from build123d import *

# Parameters (mm, degrees)
SKETCH3_R           = 73.025
BOSS_EXTRUDE2_DEPTH = 3.175
SKETCH5_R           = 31.75
CUT_EXTRUDE3_DEPTH  = 7.35
CUT_EXTRUDE4_DEPTH  = 7.35
SKETCH7_3_R         = 12.7
BOSS_EXTRUDE4_DEPTH = 3.175


with BuildPart() as part:
    # Sketch3 → Boss-Extrude2 (new body, symmetric)
    with BuildSketch(Plane.XY):
        Circle(SKETCH3_R)
    extrude(amount=BOSS_EXTRUDE2_DEPTH, both=True)

    # Sketch5 → Cut-Extrude3 (cut, through all)
    with BuildSketch(Plane.XY.offset(3.175)):
        with Locations((92.075, 0)):
            Circle(SKETCH5_R)
        with Locations((46.0375, -79.739289053)):
            Circle(SKETCH5_R)
        with Locations((-46.0375, -79.739289053)):
            Circle(SKETCH5_R)
        with Locations((-92.075, 0)):
            Circle(SKETCH5_R)
        with Locations((-46.0375, 79.739289053)):
            Circle(SKETCH5_R)
        with Locations((46.0375, 79.739289053)):
            Circle(SKETCH5_R)
        with BuildLine():
            Line((66.176953095, 30.874933265), (36.170567884, 13.550738686))
            ThreePointArc((36.170567884, 13.550738686), (27.49630657, 15.875), (29.820567884, 24.549261314))
            Line((29.820567884, 24.549261314), (59.826953095, 41.873455893))
            ThreePointArc((59.826953095, 41.873455893), (68.501214409, 39.549194579), (66.176953095, 30.874933265))
        make_face()
        with BuildLine():
            Line((59.826953095, -41.873455893), (29.820567884, -24.549261314))
            ThreePointArc((29.820567884, -24.549261314), (27.49630657, -15.875), (36.170567884, -13.550738686))
            Line((36.170567884, -13.550738686), (66.176953095, -30.874933265))
            ThreePointArc((66.176953095, -30.874933265), (68.501214409, -39.549194579), (59.826953095, -41.873455893))
        make_face()
        with BuildLine():
            Line((-6.35, -72.748389157), (-6.35, -38.1))
            ThreePointArc((-6.35, -38.1), (0, -31.75), (6.35, -38.1))
            Line((6.35, -38.1), (6.35, -72.748389157))
            ThreePointArc((6.35, -72.748389157), (0, -79.098389157), (-6.35, -72.748389157))
        make_face()
        with BuildLine():
            Line((-66.176953095, -30.874933265), (-36.170567884, -13.550738686))
            ThreePointArc((-36.170567884, -13.550738686), (-27.49630657, -15.875), (-29.820567884, -24.549261314))
            Line((-29.820567884, -24.549261314), (-59.826953095, -41.873455893))
            ThreePointArc((-59.826953095, -41.873455893), (-68.501214409, -39.549194579), (-66.176953095, -30.874933265))
        make_face()
        with BuildLine():
            Line((-59.826953095, 41.873455893), (-29.820567884, 24.549261314))
            ThreePointArc((-29.820567884, 24.549261314), (-27.49630657, 15.875), (-36.170567884, 13.550738686))
            Line((-36.170567884, 13.550738686), (-66.176953095, 30.874933265))
            ThreePointArc((-66.176953095, 30.874933265), (-68.501214409, 39.549194579), (-59.826953095, 41.873455893))
        make_face()
        with BuildLine():
            Line((6.35, 72.748389157), (6.35, 38.1))
            ThreePointArc((6.35, 38.1), (0, 31.75), (-6.35, 38.1))
            Line((-6.35, 38.1), (-6.35, 72.748389157))
            ThreePointArc((-6.35, 72.748389157), (0, 79.098389157), (6.35, 72.748389157))
        make_face()
    extrude(amount=-CUT_EXTRUDE3_DEPTH, mode=Mode.SUBTRACT)

    # Sketch7 → Cut-Extrude4 (cut, through all)
    with BuildSketch(Plane.XY.offset(3.175)):
        with BuildLine():
            Line((6.148361062, 1.5875), (7.735861062, 1.5875))
            Line((7.735861062, 1.5875), (7.735861062, -1.5875))
            Line((7.735861062, -1.5875), (6.148361062, -1.5875))
            ThreePointArc((6.148361062, -1.5875), (-6.35, 0), (6.148361062, 1.5875))
        make_face()
    extrude(amount=-CUT_EXTRUDE4_DEPTH, mode=Mode.SUBTRACT)

    # Sketch7_3 → Boss-Extrude4 (add)
    with BuildSketch(Plane.XY.offset(3.175)):
        Circle(SKETCH7_3_R)
        with BuildLine():
            Line((6.148361062, 1.5875), (7.735861062, 1.5875))
            Line((7.735861062, 1.5875), (7.735861062, -1.5875))
            Line((7.735861062, -1.5875), (6.148361062, -1.5875))
            ThreePointArc((6.148361062, -1.5875), (-6.35, 0), (6.148361062, 1.5875))
        make_face(mode=Mode.SUBTRACT)
    extrude(amount=BOSS_EXTRUDE4_DEPTH)


solid = part.part
Geometry check sheet. Reference: the model listing, model coordinates, mm. A direction names the side the tool comes from. Round coordinates to 2 decimals unless told otherwise and drop trailing zeros. Loops run counter-clockwise (first coordinate to the right, second up) from the corner with the lowest first, then second, coordinate; pieces in that order, holes last. Notation, with made-up numbers: (2.5, -19) -> (9.5, -19) arc R33 ccw to (9.5, 15) -> close; hole circle Ø7 at (19, -22). An arc over 180 degrees is marked (long way). Answer as a JSON object with one key per item and string values. Group by question number.
Item 1: Cross-section at D-D, the plane y = -54. Record the cut outline in (x, z) (3 decimals), plus the area to 3 significant figures.
Item 2: Release check for a two-part mould opening along X. For faces 4 (the face through (6.35, 56, 0)), 5 (the face through (10.964, 72.197, 0.044)), 6 (the face through (-57.043, 45.593, 0.044)) record: pulls with the +X half, pulls with the -X half, needs draft (parallel to the pull), parting line crosses it, or undercut.
Item 3: Thickness scan on line 1 along X through (y, z) = (0, 3) (3 decimals); line 2 along Y through (x, z) = (-51, 0); line 3 along Y through (x, z) = (-47, 1.75). Record the ranges inside material, lowest first.
Item 4: Set-up check for faces 1 (the face through (6.35, -55, 0)), 2 (the face through (-6.35, 55, 0)), 3 (the face through (45.03, -33.33, 0.04)): record each of +Z, -Z, +X, -X, +Y, -Y from which the full face is reachable in a straight line by a thin tool's end or side.
Item 5: Cross-section at C-C, the plane x = -38.5. Record the cut outline in (y, z) (3 decimals), plus the area to 3 significant figures.
Item 6: Depth check by flat-ended pin: pin 1 Ø4 at (y, z) = (14.5, 4.5) entering from -X; pin 2 Ø3 at (y, z) = (53, -1) entering from -X; pin 3 Ø4 at (x, z) = (40, 4.5) entering from +Y; pin 4 Ø11.5 at (x, y) = (0, 0) entering from +Z. Enter the tip coordinate at first touch or a pass-through.
Item 7: Cross-section at B-B, the plane y = -19.05. Record the cut outline in (x, z) (3 decimals), plus the area to 3 significant figures.
Item 8: Cross-section at A-A, the plane x = 0. Record the cut outline in (y, z) (3 decimals).
Determined:
{
 "1": {"outline": "(-27.448, -3.175) -> (-6.35, -3.175) -> (-6.35, 3.175) -> (-27.448, 3.175) -> close; (6.35, -3.175) -> (27.448, -3.175) -> (27.448, 3.175) -> (6.35, 3.175) -> close", "area": "268 mm²"},
 "2": {"face 4": "undercut", "face 5": "pulls with the +X half", "face 6": "pulls with the -X half"},
 "3": {"line 1": "x = -60.325 to -6.35, 7.736 to 60.325", "line 2": "y = -48.38 to -36.78, -22.11 to 22.11, 36.78 to 48.38", "line 3": "y = -48 to -34.47, -19.8 to 19.8, 34.47 to 48"},
 "4": {"face 1": "+Z, -Z, -Y", "face 2": "+Z, -Z, +Y", "face 3": "+Z, -Z"},
 "5": {"outline": "(-48.897, -3.175) -> (-29.56, -3.175) -> (-29.56, 3.175) -> (-48.897, 3.175) -> close; (-14.896, -3.175) -> (14.896, -3.175) -> (14.896, 3.175) -> (-14.896, 3.175) -> close; (29.56, -3.175) -> (48.897, -3.175) -> (48.897, 3.175) -> (29.56, 3.175) -> close", "area": "435 mm²"},
 "6": {"pin 1": "stops at x = -64.65", "pin 2": "stops at x = -31.53", "pin 3": "stops at y = 48.9", "pin 4": "passes through"},
 "7": {"outline": "(-66.675, -3.175) -> (-45.696, -3.175) -> (-45.696, 3.175) -> (-66.675, 3.175) -> close; (-26.646, -3.175) -> (26.646, -3.175) -> (26.646, 3.175) -> (-26.646, 3.175) -> close; (45.696, -3.175) -> (66.675, -3.175) -> (66.675, 3.175) -> (45.696, 3.175) -> close", "area": "605 mm²"},
 "8": {"outline": "(-31.75, -3.175) -> (-6.35, -3.175) -> (-6.35, 6.35) -> (-12.7, 6.35) -> (-12.7, 3.175) -> (-31.75, 3.175) -> close; (6.35, -3.175) -> (31.75, -3.175) -> (31.75, 3.175) -> (12.7, 3.175) -> (12.7, 6.35) -> (6.35, 6.35) -> close"}
}
